Build history of the part. All positions in model axes, mm. Give positions to 0.01 mm unless a question says otherwise; leave off trailing zeros. Loops run counter-clockwise (first coordinate to the right, second up) from the corner with the lowest first, then second, coordinate; pieces in that order, holes last. Notation, with made-up numbers: (34.5, -20) -> (44.5, -20) arc R20 ccw to (44.5, -10) -> close; hole circle Ø9 at (-7, 0.5). An arc over 180 degrees is marked (long way). One line per question, with ' | ' between items. Start each with the question number.
(1) Slice it at D-D, the plane z = 2.15. Give the number of separate pieces and of enclosed holes in the cut face, then the cut area to 3 significant figures.
(2) Flat gauge pins, fed straight in: pin 1 Ø1 at (y, z) = (110, 2) entering from -X; pin 2 Ø1.4 at (x, z) = (5.5, 1.5) entering from +Y; pin 3 Ø3.5 at (x, y) = (-49, 105) entering from -Z; pin 4 Ø1.4 at (x, z) = (-82.5, 2.5) entering from -Y. Where does each tip first touch, or does it go through?
(3) Slice it at A-A, the plane x = -39. Write the cut outline in (y, z), then the cut area to 3 significant figures.
(4) Slice it at B-B, the plane x = -49. Write the cut outline in (y, z), then the cut area to 3 significant figures.
(5) Drill centre lines: L1, parallel to Y at x = -29, z = 2.5; L2, parallel to Y at x = -2.5, z = 0.9; L3, parallel to Y at x = -39, z = 2.5. Where is each one in solid material? Low to high. Write a range as from..to.
(6) Slice it at C-C, the plane y = 78. Write the cut outline in (x, z).
```python
from build123d import *

# Parameters (mm, degrees)
MODEL_R                  = 1.6
MODEL_R_2                = 2
MODEL_R_3                = 5.5
RESSALTO_EXTRUS_O1_DEPTH = 5


with BuildPart() as part:
    # Model → Ressalto-extrusão1 (new body)
    with BuildSketch(Plane.XY):
        Polygon((-6.199999159, 114.700001655), (-6.199999159, 113.500001714), (-7.999999159, 113.500001714), (-7.999999159, 110.500001669), (-6.199999159, 110.500001669), (-6.199999159, 109.300001727), (-3.799999815, 109.300001727), (-3.799999815, 110.500001669), (3.000000179, 110.500001669), (3.000000179, 108.000001654), (7.500000924, 108.000001654), (7.500000924, 103.000001535), (3.000000179, 103.000001535), (3.000000179, 100.00000149), (-3.999999195, 100.00000149), (-3.999999195, 90.000001341), (3.000000179, 90.000001341), (3.000000179, 87.000001296), (7.500000924, 87.000001296), (7.500000924, 79.000001177), (3.000000179, 79.000001177), (3.000000179, 71.000001058), (-80.999999166, 71.000001058), (-80.999999166, 79.000001177), (-85.499999911, 79.000001177), (-85.499999911, 87.000001296), (-80.999999166, 87.000001296), (-80.999999166, 90.000001341), (-73.999999791, 90.000001341), (-73.999999791, 100.00000149), (-80.999999166, 100.00000149), (-80.999999166, 103.000001535), (-85.499999911, 103.000001535), (-85.499999911, 108.000001654), (-80.999999166, 108.000001654), (-80.999999166, 110.500001669), (-74.199999172, 110.500001669), (-74.199999172, 109.300001727), (-71.799999827, 109.300001727), (-71.799999827, 110.500001669), (-69.999999827, 110.500001669), (-69.999999827, 113.500001714), (-71.799999827, 113.500001714), (-71.799999827, 114.700001655), (-74.199999172, 114.700001655), (-74.199999172, 113.500001714), (-80.999999166, 113.500001714), (-80.999999166, 120.000001773), (3.000000179, 120.000001773), (3.000000179, 113.500001714), (-3.799999815, 113.500001714), (-3.799999815, 114.700001655), align=None)
        with Locations((-38.999999449, 85.500001416)):
            Circle(MODEL_R, mode=Mode.SUBTRACT)
        with Locations((-29.000000507, 105.000001535)):
            Circle(MODEL_R_2, mode=Mode.SUBTRACT)
        with Locations((-38.999999449, 104.500001416)):
            Circle(MODEL_R, mode=Mode.SUBTRACT)
        with Locations((-49.000000507, 85.000001296)):
            Circle(MODEL_R_2, mode=Mode.SUBTRACT)
        with Locations((-49.000000507, 105.000001535)):
            Circle(MODEL_R_2, mode=Mode.SUBTRACT)
        with Locations((-38.999999493, 95.000001416)):
            Circle(MODEL_R_3, mode=Mode.SUBTRACT)
        with Locations((-29.000000507, 85.000001296)):
            Circle(MODEL_R_2, mode=Mode.SUBTRACT)
    extrude(amount=RESSALTO_EXTRUS_O1_DEPTH)


solid = part.part
```
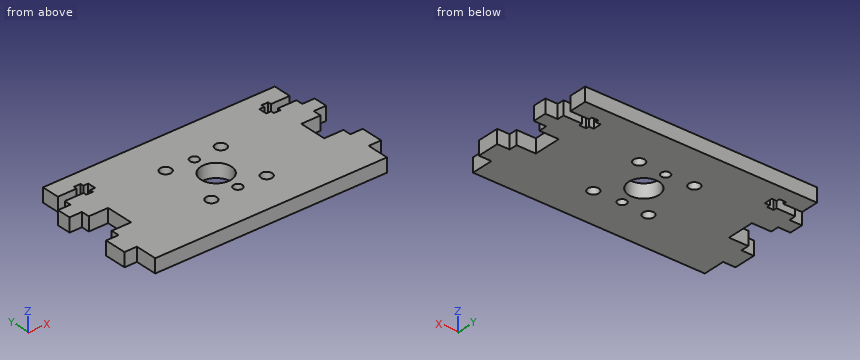
Final values:
1) separate pieces: 1 | enclosed holes: 7 | area: 3,850 mm2
2) pin 1: x = -81 | pin 2: y = 108 | pin 3: through | pin 4: y = 79
3) outline: (71, 0) -> (83.9, 0) -> (83.9, 5) -> (71, 5) -> close; (87.1, 0) -> (89.5, 0) -> (89.5, 5) -> (87.1, 5) -> close; (100.5, 0) -> (102.9, 0) -> (102.9, 5) -> (100.5, 5) -> close; (106.1, 0) -> (120, 0) -> (120, 5) -> (106.1, 5) -> close | area: 158 mm2
4) outline: (71, 0) -> (83, 0) -> (83, 5) -> (71, 5) -> close; (87, 0) -> (103, 0) -> (103, 5) -> (87, 5) -> close; (107, 0) -> (120, 0) -> (120, 5) -> (107, 5) -> close | area: 205 mm2
5) L1: 71..83, 87..103, 107..120 | L2: 71..90, 100..110.5, 113.5..120 | L3: 71..83.9, 87.1..89.5, 100.5..102.9, 106.1..120
6) outline: (-81, 0) -> (3, 0) -> (3, 5) -> (-81, 5) -> close
